```python
from build123d import *

# Parameters (mm, degrees)
BOSS_EXTRUDE1_DEPTH                                 = 24
SKETCH2_W                                           = 151
SKETCH2_H                                           = 56
CUT_EXTRUDE1_DEPTH                                  = 22
SKETCH3_W                                           = 156
SKETCH3_H                                           = 61
CUT_EXTRUDE2_DEPTH                                  = 5
SKETCH4_R                                           = 6.5
SKETCH4_R_2                                         = 4
SKETCH4_W                                           = 98
SKETCH4_H                                           = 40.5
CUT_EXTRUDE3_DEPTH                                  = 4
CBORE_FOR_M4_HEX_SOCKET_HEAD_CAP_SCREW1_D           = 4.5
CBORE_FOR_M4_HEX_SOCKET_HEAD_CAP_SCREW1_CBORE_D     = 8
CBORE_FOR_M4_HEX_SOCKET_HEAD_CAP_SCREW1_CBORE_DEPTH = 4.4
SKETCH7_W                                           = 6.5
SKETCH7_H                                           = 6.5
BOSS_EXTRUDE2_DEPTH                                 = 11
F_2_0MM_DOWEL_HOLE1_D                               = 2
F_2_0MM_DOWEL_HOLE1_DEPTH                           = 8
F_2_0MM_DOWEL_HOLE1_TIP                             = 0.600860619
SKETCH13_W                                          = 15
SKETCH13_H                                          = 20
CUT_EXTRUDE6_DEPTH                                  = 24
SKETCH14_W                                          = 6
SKETCH14_H                                          = 31
CUT_EXTRUDE7_DEPTH                                  = 3


with BuildPart() as part:
    # Sketch1 → Boss-Extrude1 (new body)
    with BuildSketch(Plane.XY):
        Polygon((-93, 10.5), (-78, 10.5), (-78, -30.5), (78, -30.5), (78, 10.5), (93, 10.5), (93, 30.5), (-93, 30.5), align=None)
    extrude(amount=BOSS_EXTRUDE1_DEPTH)

    # Sketch2 → Cut-Extrude1 (cut)
    with BuildSketch(Plane(origin=(0, 0, 0), x_dir=(-1, 0, 0), z_dir=(0, 0, -1))):
        Rectangle(SKETCH2_W, SKETCH2_H)
    extrude(amount=-CUT_EXTRUDE1_DEPTH, mode=Mode.SUBTRACT)

    # Sketch3 → Cut-Extrude2 (cut)
    with BuildSketch(Plane(origin=(0, 0, 0), x_dir=(-1, 0, 0), z_dir=(0, 0, -1))):
        Rectangle(SKETCH3_W, SKETCH3_H)
    extrude(amount=-CUT_EXTRUDE2_DEPTH, mode=Mode.SUBTRACT)

    # Sketch4 → Cut-Extrude3 (cut)
    with BuildSketch(Plane.XY.offset(24)):
        with Locations((61.2, 17)):
            Circle(SKETCH4_R)
        with Locations((62.3, -1.25)):
            Circle(SKETCH4_R_2)
        with Locations((61.7, -19.3)):
            Circle(SKETCH4_R_2)
        with Locations((-12.7, -5.45)):
            Rectangle(SKETCH4_W, SKETCH4_H)
    extrude(amount=-CUT_EXTRUDE3_DEPTH, mode=Mode.SUBTRACT)

    # CBORE for M4 Hex Socket Head Cap Screw1 (through all)
    with Locations(Plane.XY.offset(24)):
        with Locations((-85, 20.5), (85, 20.376125295)):
            CounterBoreHole(CBORE_FOR_M4_HEX_SOCKET_HEAD_CAP_SCREW1_D / 2, CBORE_FOR_M4_HEX_SOCKET_HEAD_CAP_SCREW1_CBORE_D / 2, CBORE_FOR_M4_HEX_SOCKET_HEAD_CAP_SCREW1_CBORE_DEPTH)

    # Sketch7 → Boss-Extrude2 (add)
    with BuildSketch(Plane(origin=(0, 0, 22), x_dir=(-1, 0, 0), z_dir=(0, 0, -1))):
        with Locations((-72.25, 24.75)):
            Rectangle(SKETCH7_W, SKETCH7_H)
        with Locations((-72.25, -24.75)):
            Rectangle(SKETCH7_W, SKETCH7_H)
        with Locations((72.25, 24.75)):
            Rectangle(SKETCH7_W, SKETCH7_H)
        with Locations((72.25, -24.75)):
            Rectangle(SKETCH7_W, SKETCH7_H)
    extrude(amount=BOSS_EXTRUDE2_DEPTH)

    # Ø2.0mm Dowel Hole1
    with Locations(Plane(origin=(0, 0, 11), x_dir=(-1, 0, 0), z_dir=(0, 0, -1))):
        with Locations((-72.25, 24.75), (-72.25, -24.75), (72.25, 24.75), (72.25, -24.75)):
            Hole(F_2_0MM_DOWEL_HOLE1_D / 2, depth=F_2_0MM_DOWEL_HOLE1_DEPTH)
            with Locations((0, 0, -(F_2_0MM_DOWEL_HOLE1_DEPTH + F_2_0MM_DOWEL_HOLE1_TIP / 2))):  # 118° drill point
                Cone(0, F_2_0MM_DOWEL_HOLE1_D / 2, F_2_0MM_DOWEL_HOLE1_TIP, mode=Mode.SUBTRACT)

    # Sketch13 → Cut-Extrude6 (cut)
    with BuildSketch(Plane(origin=(0, 0, 0), x_dir=(-1, 0, 0), z_dir=(0, 0, -1))):
        with Locations((-85.5, 20.5)):
            Rectangle(SKETCH13_W, SKETCH13_H)
        with Locations((85.5, 20.5)):
            Rectangle(SKETCH13_W, SKETCH13_H)
    extrude(amount=-CUT_EXTRUDE6_DEPTH, mode=Mode.SUBTRACT)

    # Sketch14 → Cut-Extrude7 (cut)
    with BuildSketch(Plane.ZY.offset(78)):
        with Locations((8, -6)):
            Rectangle(SKETCH14_W, SKETCH14_H)
    extrude(amount=-CUT_EXTRUDE7_DEPTH, mode=Mode.SUBTRACT)


solid = part.part
```
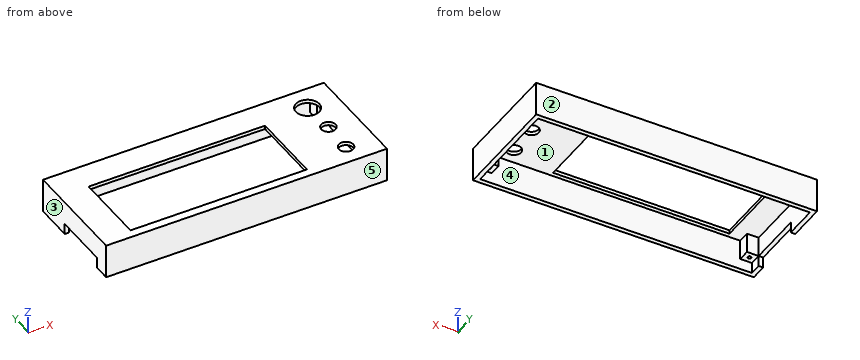
For this review, take the finished solid that the model builds, in its own axes (mm). Face numbers are marked on the shaded views. A direction names the side the tool comes from. Give positions to 0.01 mm unless a question says otherwise; leave off trailing zeros. Write each loop counter-clockwise with the first axis right and the second up, starting at its lowest first coordinate (ties: lowest second). Pieces come first, ordered by that corner, then holes.
Item 1: Insertion check: P1, Ø8, axis at x = -17.5, y = 21.5, coming from the -Z side; P2, Ø2.5, axis at x = -72.25, y = 24.75, coming from the -Z side. Each pin has a flat end and moves straight along its axis. Give the tip position at first contact, or say it passes through.
Item 2: Take a section at B-B (x = 22). Give the boundary of the cut face in (y, z), and give its area (3 significant figures).
Item 3: Take a section at C-C (z = 14.5). Give the boundary of the cut face in (x, y), and give its area (3 significant figures).
Item 4: Wall thickness on probe 1 along X at (y, z) = (-24.75, 13.5); probe 2 along Y at (x, z) = (-34.5, 19.75); probe 3 along X at (y, z) = (-21, 14.5): over which ranges is each line inside the solid? List them lowest first.
Item 5: Machinability: for the marked faces 1 and 2, which of the approach directions +Z, -Z, +X, -X, +Y, -Y give a long, thin tool a straight path to every point of the face, cutting with its end or side? Answer none if there is none.
Item 6: Take a section at D-D (x = 62.3). Give the boundary of the cut face in (y, z).
Item 7: The part is to be moulded in two halves that separate along Y. For the marked faces 3, 4 and 5, say which applies: +Y half, -Y half, draft (parallel to the pull), parting line (faces both ways), or undercut.
Item 8: Take a section at A-A (y = -12). Give the boundary of the cut face in (x, z), and give its area (3 significant figures).
Established:
1. P1: stops at z = 22
1. P2: stops at z = 11
2. outline: (-30.5, 5) - (-28, 5) - (-28, 22) - (-25.7, 22) - (-25.7, 24) - (-30.5, 24) - close; (14.8, 22) - (28, 22) - (28, 5) - (30.5, 5) - (30.5, 24) - (14.8, 24) - close
2. area: 126 mm2
3. outline: (-78, -30.5) - (78, -30.5) - (78, 30.5) - (-78, 30.5) - close; hole (-75.5, -21.5) - (-69, -21.5) - (-69, -28) - (69, -28) - (69, -21.5) - (75.5, -21.5) - (75.5, 21.5) - (69, 21.5) - (69, 28) - (-69, 28) - (-69, 21.5) - (-75.5, 21.5) - close; hole circle Ø2 at (-72.25, -24.75); hole circle Ø2 at (-72.25, 24.75); hole circle Ø2 at (72.25, -24.75); hole circle Ø2 at (72.25, 24.75)
3. area: 1,220 mm2
4. probe 1: x = -78 to -73.25, -71.25 to -69, 69 to 71.25, 73.25 to 78
4. probe 2: y = -30.5 to -28, 28 to 30.5
4. probe 3: x = -78 to -75.5, 75.5 to 78
5. face 1: -Z
5. face 2: +Z, -Z, +X, -X, +Y
6. outline: (-30.5, 5) - (-28, 5) - (-28, 22) - (-23.25, 22) - (-23.25, 24) - (-30.5, 24) - close; (-15.35, 22) - (-5.25, 22) - (-5.25, 24) - (-15.35, 24) - close; (2.75, 22) - (10.59, 22) - (10.59, 24) - (2.75, 24) - close; (23.41, 22) - (28, 22) - (28, 5) - (30.5, 5) - (30.5, 24) - (23.41, 24) - close
7. face 3: draft
7. face 4: undercut
7. face 5: -Y half
8. outline: (-78, 11) - (-75.5, 11) - (-75.5, 22) - (-61.7, 22) - (-61.7, 24) - (-78, 24) - close; (36.3, 22) - (75.5, 22) - (75.5, 5) - (78, 5) - (78, 24) - (36.3, 24) - close
8. area: 186 mm2
